```python
from build123d import *

# Parameters (mm, degrees)
F1_DEPTH = 34.1249
F5_DEPTH = 0.5
F7_DEPTH = 0.5
F9_DEPTH = 1


with BuildPart() as f1:
    # F0 (on Right) → F1 (new body, symmetric)
    with BuildSketch(Plane.YZ):
        Polygon((-13.4874, 0), (0, 0), (13.4874, 0), (13.4874, 28.575), (0, 28.575), (-13.4874, 28.575), align=None)
    extrude(amount=F1_DEPTH, both=True)

    # F4 (on offset) → F5 (join)
    with BuildSketch(Plane.XY.offset(6)):
        with BuildLine():
            ThreePointArc((-2, -19.22551), (0, -21.22551), (2, -19.22551))
            ThreePointArc((2, -19.22551), (0, -17.22551), (-2, -19.22551))
        make_face()
        with BuildLine():
            ThreePointArc((-2, -19.22551), (0, -17.22551), (2, -19.22551))
            Line((2, -19.22551), (2, 0))
            Line((2, 0), (-2, 0))
            Line((-2, 0), (-2, -19.22551))
        make_face()
        with BuildLine():
            ThreePointArc((-14.265118, -19.22551), (-12.265118, -21.22551), (-10.265118, -19.22551))
            ThreePointArc((-10.265118, -19.22551), (-12.265118, -17.22551), (-14.265118, -19.22551))
        make_face()
        with BuildLine():
            ThreePointArc((-14.265118, -19.22551), (-12.265118, -17.22551), (-10.265118, -19.22551))
            Line((-10.265118, -19.22551), (-10.265118, 0))
            Line((-10.265118, 0), (-14.265118, 0))
            Line((-14.265118, 0), (-14.265118, -19.22551))
        make_face()
        with BuildLine():
            ThreePointArc((8.530043, -19.22551), (10.530043, -21.22551), (12.530043, -19.22551))
            ThreePointArc((12.530043, -19.22551), (10.530043, -17.22551), (8.530043, -19.22551))
        make_face()
        with BuildLine():
            ThreePointArc((8.530043, -19.22551), (10.530043, -17.22551), (12.530043, -19.22551))
            Line((12.530043, -19.22551), (12.530043, 0))
            Line((12.530043, 0), (8.530043, 0))
            Line((8.530043, 0), (8.530043, -19.22551))
        make_face()
    extrude(amount=F5_DEPTH)

    # F6 (on offset) → F7 (join)
    with BuildSketch(Plane.XY.offset(25)):
        with BuildLine():
            ThreePointArc((8.530043, -19.22551), (10.530043, -21.22551), (12.530043, -19.22551))
            Line((12.530043, -19.22551), (12.530043, -13.4874))
            Line((12.530043, -13.4874), (8.530043, -13.4874))
            Line((8.530043, -13.4874), (8.530043, -19.22551))
        make_face()
        with BuildLine():
            ThreePointArc((-2, -19.22551), (0, -21.22551), (2, -19.22551))
            Line((2, -19.22551), (2, -13.4874))
            Line((2, -13.4874), (-2, -13.4874))
            Line((-2, -13.4874), (-2, -19.22551))
        make_face()
        with BuildLine():
            ThreePointArc((-14.265118, -19.22551), (-12.265118, -21.22551), (-10.265118, -19.22551))
            Line((-10.265118, -19.22551), (-10.265118, -13.4874))
            Line((-10.265118, -13.4874), (-14.265118, -13.4874))
            Line((-14.265118, -13.4874), (-14.265118, -19.22551))
        make_face()
    extrude(amount=F7_DEPTH)

    # F8 (on Top) → F9 (join)
    with BuildSketch(Plane.XY):
        Polygon((-29.149349, 7.008), (-34.1249, 7.008), (-34.1249, -7.009424), (-28.291495, -7.009424), align=None)
        with BuildLine():
            Line((-34.1249, -7.009424), (-34.1249, 7.008))
            Line((-34.1249, 7.008), (-41.854384, 7.008))
            ThreePointArc((-41.854384, 7.008), (-37.319332, 4.732924), (-35.491192, 0))
            ThreePointArc((-35.491192, 0), (-37.324363, -4.738458), (-41.869275, -7.009424))
            Line((-41.869275, -7.009424), (-34.1249, -7.009424))
        make_face()
        with BuildLine():
            ThreePointArc((-35.491192, 0), (-37.319332, 4.732924), (-41.854384, 7.008))
            ThreePointArc((-41.854384, 7.008), (-49.57253, 0.007479), (-41.869275, -7.009424))
            ThreePointArc((-41.869275, -7.009424), (-37.324363, -4.738458), (-35.491192, 0))
        make_face()
    extrude(amount=F9_DEPTH)


solid = f1.part
```
Check sheet for the modelled part. Datum: model origin and axes. Units: mm. A direction names the side the tool comes from. Round coordinates to 2 decimals unless told otherwise and drop trailing zeros. Order: outer loops, then holes, each group sorted by start corner. A loop starts at its lowest first (then second) coordinate and runs counter-clockwise, first axis right, second up. Notation, with made-up numbers: (73, 72.5) -> (112, 72.5) arc R17 cw to (112, 99.5) -> close; hole circle Ø3 at (9, 51.25). An arc over 180 degrees is marked (long way). One line per item, written item: value. Start each with the question number.
Q1. Cross-section at D-D (y = 5). Record the boundary of the cut face in (x, z) (3 decimals), and give its area (3 significant figures).
Q2. Cross-section at C-C (z = 26.75). Record the boundary of the cut face in (x, y), and give its area (3 significant figures).
Q3. Thickness scan on line 1 (Z direction, x = 10, y = -16.5); line 2 (Y direction, x = 17.5, z = 25); line 3 (X direction, y = 11, z = 4). Record the ranges inside material, lowest first.
Q4. Cross-section at B-B (x = 0). Record the boundary of the cut face in (y, z) (1 decimal), and give its area (3 significant figures).
Q5. Mould release check, pull along X, two halves, no side actions. Record for faces 1 (the face through (-12.309, -21.225, 6.246)), 2 (the face through (34.125, 0, 14)), 3 (the face through (-42, 0, 1)): pulls with the +X half, pulls with the -X half, needs draft (parallel to the pull), parting line crosses it, or undercut.
Q6. Set-up check for faces 4 (the face through (-12, -17, 25.5)), 5 (the face through (-12.309, -21.225, 25.246)), 6 (the face through (-12, -17, 6)), 7 (the face through (-12, -17, 25)): record each of +Z, -Z, +X, -X, +Y, -Y from which the full face is reachable in a straight line by a thin tool's end or side.
Q7. Gauge pin test, flat ends, axial feed: pin 1 Ø0.8 at (x, z) = (-37.5, 0.5) entering from +Y; pin 2 Ø4.5 at (x, y) = (-11.5, -16.5) entering from -Z; pin 3 Ø10 at (x, z) = (-30, 17.5) entering from -Y. Record the tip position at first contact, or that the pin passes through.
Q8. Cross-section at A-A (y = 0). Record the boundary of the cut face in (x, z) (3 decimals).
Completed:
1. outline: (-47.489, 0) -> (34.125, 0) -> (34.125, 28.575) -> (-34.125, 28.575) -> (-34.125, 1) -> (-47.489, 1) -> close
1. area: 1,960 mm²
2. outline: (-34.12, -13.49) -> (34.12, -13.49) -> (34.12, 13.49) -> (-34.12, 13.49) -> close
2. area: 1,840 mm²
3. line 1: z = 6 to 6.5, 25 to 25.5
3. line 2: y = -13.49 to 13.49
3. line 3: x = -34.12 to 34.12
4. outline: (-21.2, 6) -> (-13.5, 6) -> (-13.5, 0) -> (13.5, 0) -> (13.5, 28.6) -> (-13.5, 28.6) -> (-13.5, 25.5) -> (-21.2, 25.5) -> (-21.2, 25) -> (-13.5, 25) -> (-13.5, 6.5) -> (-21.2, 6.5) -> close
4. area: 779 mm²
5. face 1: undercut
5. face 2: pulls with the +X half
5. face 3: needs draft
6. face 4: +Z, +X, -X, -Y
6. face 5: +Z, -Z, -Y
6. face 6: -Z, +X, -X, -Y
6. face 7: +X, -X, -Y
7. pin 1: stops at y = 7.01
7. pin 2: stops at z = 6
7. pin 3: stops at y = -13.49
8. outline: (-49.573, 0) -> (34.125, 0) -> (34.125, 28.575) -> (-34.125, 28.575) -> (-34.125, 1) -> (-49.573, 1) -> close
